Autodesk Inventor part; units mm, degrees
ref_plane "Work Plane1" through (0, -5, 0) normal (0, 1, 0) x (-1, 0, 0)
ref_plane "YZ Plane" through (0, 0, 0) normal (1, 0, 0) x (0, 1, 0)
ref_plane "XY Plane" through (0, 0, 0) normal (0, 0, 1) x (1, 0, 0)
sketch "Sketch1" plane through (0, 0, 0) normal (0, 0, 1) x (1, 0, 0)
  line L0 (0, 60) -> (25, 8)
  line L1 (25, 8) -> (0, -5)
  line L2 (0, -5) -> (0, 0)
  line L3 (0, 0) -> (0, 60)
  dimension "d1" = 60
  dimension "d2" = 13
  dimension "d18" = 5
  dimension "d19" = 25
revolve "Revolution1" add sketch "Sketch1" angle 360 about axis through (0, 0, 0) along (0, 1, 0)
ref_plane "Work Plane1" through (0, -5, 0) normal (0, 1, 0) x (-1, 0, 0)
sketch "Sketch3" plane through (0, -5, 0) normal (0, 1, 0) x (-1, 0, 0)
  circle A0 centre (0, 0) radius 25
  circle A1 centre (0, 0) radius 41.25
  dimension "d7" = 50
  dimension "d8" = 82.5
extrude "Extrusion1" add sketch "Sketch3" against normal blind 8
sketch "Sketch4" plane through (0, 0, 0) normal (0, 0, 1) x (1, 0, 0)
  line L0 (0, 60) -> (-25, 8)
  line L1 (41.25, -5) -> (-41.25, -5)
  line L2 (-25, -13) -> (-25, -5)
  line L3 (25, -13) -> (25, -5)
  line L4 (41.25, -5) -> (41.25, -13)
  line L5 (-41.25, -5) -> (-41.25, -13)
  line L6 (25, 8) -> (0, -5)
  line L7 (0, 60) -> (25, 8)
  line L8 (-37.2957, -1.4547) -> (-41.25, -5)
  line L9 (-25, -5) -> (-15.8228, 3.2278)
  line L10 (-41.25, -5) -> (-25, -5)
  line L11 (-25, 8) -> (25, 8)
  line L12 (-25, 8) -> (-12.5712, 19.143)
  line L13 (-12.5712, 19.143) -> (-7.4345, 10.7484)
  line L14 (-7.4345, 10.7484) -> (-15.8228, 3.2278)
  line L15 (-25, 8) -> (-30.5847, -1.4547)
  line L16 (-37.2957, -1.4547) -> (-30.5847, -1.4547)
  point P0 (0, 0)
  point P1 (0, -5)
  point P2 (-10.5, 8)
extrude "Extrusion2" add sketch "Sketch4" along normal mid plane 5 contours L11 L14 L9 L1 L8 L16 L15
pattern_circular "Circular Pattern1" count 3 over 360 about axis through (0, -10, 0) along (0, 1, 0) of "Extrusion2"
sketch "Sketch5" plane through (0, -5, 0) normal (0, 1, 0) x (1, 0, 0)
  circle A0 centre (0, 0) radius 39.5
  circle A1 centre (0, 0) radius 28.5
  dimension "d16" = 79
  dimension "d17" = 57
sketch "Sketch6" plane through (0, -5, 0) normal (0, 1, 0) x (1, 0, 0)
  circle A0 centre (0, 0) radius 41.25
  circle A1 centre (0, 0) radius 45.75
  circle A2 centre (0, 0) radius 53.5003
  dimension "d20" = 82.5
  dimension "d21" = 4.5
extrude "Extrusion3" add sketch "Sketch6" against normal blind 8 contours A1 | A2
sketch "Sketch7" plane through (0, -5, 0) normal (0, 1, 0) x (1, 0, 0)
  circle A0 centre (0, 0) radius 45.75
  circle A1 centre (0, 0) radius 41.25
extrude "Extrusion4" cut sketch "Sketch7" against normal blind 4
sketch "Sketch8" plane through (0, -13, 0) normal (0, -1, 0) x (1, 0, 0)
  circle A0 centre (0, 0) radius 53.5003
  circle A1 centre (0, 0) radius 53.5003
  circle A2 centre (0, 0) radius 43.5003
  line L0 (0, -60.7067) -> (0, 74.3031)
  line L1 (53.5003, -65.9653) -> (53.5003, 59.8233)
  line L2 (-62.5744, 0) -> (102.4614, 0)
  line L3 (-37.8313, -65.5258) -> (42.3793, 73.4032)
  line L4 (39.8021, -68.9393) -> (-31.97, 55.3736)
  point P0 (26.7502, 46.3326)
  point P1 (21.7502, 37.6724)
  point P2 (43.5003, 0)
  point P3 (53.5003, 0)
  point P4 (-21.7502, -37.6724)
  point P5 (-26.7502, -46.3326)
  point P6 (26.7502, -46.3326)
  point P7 (21.7502, -37.6724)
  point P8 (-21.7502, 37.6724)
  point P9 (-26.7502, 46.3326)
  point P10 (-53.5003, 0)
  point P11 (-43.5003, 0)
  dimension "d26" = 0
  dimension "d27" = 10
  dimension "d28" = 120
  dimension "d29" = 120
  dimension "d30" = 120
extrude "Extrusion5" add sketch "Sketch8" along normal blind 30 contours L2 A2 L3 A0 | A0 L0 A2 L4 | A0 L3 A2 L0 | L4 A2 L2 A0 picked at (40.4215, 23.3374) picked at (5.6147, -49.6757) picked at (-3.0967, -49.896) picked at (-40.4215, 23.3374)
equation "\"d29\" = d28"
properties part number "Reflector+feet"
Work out the finished part from the listing and answer in its coordinate system (mm). A direction names the side the tool comes from. Give positions to 0.01 mm unless a question says otherwise; leave off trailing zeros. Loops run counter-clockwise (first coordinate to the right, second up) from the corner with the lowest first, then second, coordinate; pieces in that order, holes last. Notation, with made-up numbers: (7, -8) -> (26, -8) arc R25 ccw to (26, 21) -> close; hole circle Ø1 at (78, 68). An arc over 180 degrees is marked (long way). Write item = value, one per line. Start each with the question number.
(1) The mould has two halves that part along X. Classify faces 1 (the cylindrical face through (-37.831, -27.79, 21.473)), 2 (the flat face through (-40, -43, 22)), 3 (the flat face through (24.285, -27.79, -42.063)): +X half, -X half, draft (parallel to the pull), parting line (faces both ways), or undercut.
(2) Given pin 1 Ø14.5 at (x, y) = (-32.5, 4.5) entering from +Z; pin 2 Ø8 at (y, z) = (31, 11) entering from -X; pin 3 Ø14.5 at (x, y) = (-34.5, 2.5) entering from -Z; pin 4 Ø6 at (y, z) = (-24.5, -33.5) entering from -X, each flat-ended and moving along its own axis, determine where each tip first touches the part or whether it passes through.
(3) Find section A-A on y = -26. Give the vertices of the cut face in (x, z), and give its area (3 significant figures).
(4) Find the intervals of material crossed by probe 1 along Z at (x, y) = (0, -8); probe 2 along Z at (x, y) = (-20, -8.5); probe 3 along Z at (x, y) = (-35.5, -5.5), in increasing order. Write a range as from..to.
(5) Find section B-B on z = -10. Give the number of separate pieces and of enclosed holes in the cut face, and give its area (3 significant figures).
(6) Which of the six approach directions +Z, -Z, +X, -X, +Y, -Y give full straight-line access (tool end or side, diameter ignored) to faces 4 (the flat face through (-49, -28, 0)), 5 (the cylindrical face through (43.64, -6.97, -13.74)), 6 (the flat face through (25, -13, -7)), 7 (the flat face through (24.215, -27.79, 41.942)), 8 (the flat face through (-26, 0, -2.5))?
(7) Find section D-D on y = 33.5. Give the vertices of the cut face in (x, z), and give its area (3 significant figures).
From the geometry:
q1.face_1 = undercut
q1.face_2 = draft
q1.face_3 = +X half
q2.pin_1 = 2.5
q2.pin_2 = -12.94
q2.pin_3 = -2.5
q2.pin_4 = through
q3.outline = (-53.5, 0) -> (-43.5, 0) arc R43.5 cw to (-21.75, 37.67) -> (-26.75, 46.33) arc R53.5 ccw to start; (-26.75, -46.33) arc R53.5 ccw to (26.75, -46.33) -> (21.75, -37.67) arc R43.5 cw to (-21.75, -37.67) -> close; (21.75, 37.67) arc R43.5 cw to (43.5, 0) -> (53.5, 0) arc R53.5 ccw to (26.75, 46.33) -> close
q3.area = 1,520 mm^2
q4.probe_1 = -53.5..-45.75, -41.25..-25, 25..41.25, 45.75..53.5
q4.probe_2 = -49.62..-41.15, -36.08..-15, 15..36.08, 41.15..49.62
q4.probe_3 = -40.03..-28.86, -21.01..21.01, 28.86..40.03
q5.separate_pieces = 3
q5.enclosed_holes = 0
q5.area = 1,520 mm^2
q6.face_4 = -Z, +X, -X, -Y
q6.face_5 = +Y
q6.face_6 = -Y
q6.face_7 = +Z, -Y
q6.face_8 = -Z, -X
q7.outline = circle Ø25.48 at (0, 0)
q7.area = 510 mm^2
